Could you check a few things on this model? Use its own coordinates, in mm. Face numbers are marked on the shaded views. A direction names the side the tool comes from. Give positions to 0.01 mm unless a question says otherwise; leave off trailing zeros. Loops run counter-clockwise (first coordinate to the right, second up) from the corner with the lowest first, then second, coordinate; pieces in that order, holes last.
1. Imagine slicing it at A-A (z = 7.5). List the corners of the cut face in (x, y) for me, plus the area to 3 significant figures.
2. For the marked faces 1, 2, 3 and 4, which set-ups out of +Z, -Z, +X, -X, +Y, -Y let a thin tool reach every point of the face, with its end or its side?
3. Imagine slicing it at B-B (x = 7.5). List the corners of the cut face in (y, z) for me.
4. Thinking about a two-plate mould opening in X: for the marked faces 5, 6 and 7, which applies, +X half, -X half, draft (parallel to the pull), parting line (faces both ways), or undercut?
5. I need wall thicknesses on line 1 along Y through (x, z) = (-0.75, 7.25); line 2 along Y through (x, z) = (8.5, 1.5); line 3 along Y through (x, z) = (-6, 3.25). Which ranges of each line are inside material? Lowest first, please.
6. Imagine slicing it at C-C (x = 10). List the corners of the cut face in (y, z) for me, plus the area to 4 significant figures.
7. Imagine slicing it at D-D (z = 5.5). List the corners of the cut face in (x, y) for me.
8. For P1, Ø1.5, axis at y = 4, z = 6, coming from the -X side; P2, Ø3, axis at x = 9, y = 25, coming from the +Z side; P3, Ø1.2, axis at x = -5, y = 5, coming from the +Z side, each with a flat end and sliding along its axis, tell me the tip position at first contact or that it passes through.
```python
from build123d import *

# Parameters (mm, degrees)
SKETCH1_W           = 24
SKETCH1_H           = 19.5
BOSS_EXTRUDE1_DEPTH = 3
SKETCH3_W           = 19
SKETCH3_H           = 4.5
BOSS_EXTRUDE2_DEPTH = 1.5
SKETCH4_W           = 19
SKETCH4_H           = 6.5
BOSS_EXTRUDE3_DEPTH = 1.5
CUT_EXTRUDE1_DEPTH  = 1.5
SKETCH6_W           = 24
SKETCH6_H           = 3
BOSS_EXTRUDE4_DEPTH = 29.5
SKETCH7_W           = 4.5
SKETCH7_H           = 4.5
CUT_EXTRUDE2_DEPTH  = 39.373167709
CHAMFER1_SIZE       = 3


with BuildPart() as part:
    # Sketch1 → Boss-Extrude1 (new body)
    with BuildSketch(Plane(origin=(0, 0, 0), x_dir=(1, 0, 0), z_dir=(0, 1, 0))):
        Rectangle(SKETCH1_W, SKETCH1_H)
    extrude(amount=BOSS_EXTRUDE1_DEPTH)

    # Sketch3 → Boss-Extrude2 (add)
    with BuildSketch(Plane(origin=(0, 3, 0), x_dir=(1, 0, 0), z_dir=(0, 1, 0))):
        with Locations((0, -4.8)):
            Rectangle(SKETCH3_W, SKETCH3_H)
    extrude(amount=BOSS_EXTRUDE2_DEPTH)

    # Sketch4 → Boss-Extrude3 (add)
    with BuildSketch(Plane(origin=(0, 4.5, 0), x_dir=(1, 0, 0), z_dir=(0, 1, 0))):
        with Locations((0, -4.8)):
            Rectangle(SKETCH4_W, SKETCH4_H)
    extrude(amount=BOSS_EXTRUDE3_DEPTH)

    # Sketch5 → Cut-Extrude1 (cut)
    with BuildSketch(Plane(origin=(0, 6, 0), x_dir=(1, 0, 0), z_dir=(0, 1, 0))):
        Polygon((0, -2.8), (0.75, -1.55), (-0.75, -1.55), align=None)
        Polygon((0, -6.8), (0.75, -8.05), (-0.75, -8.05), align=None)
    extrude(amount=-CUT_EXTRUDE1_DEPTH, mode=Mode.SUBTRACT)

    # Sketch6 → Boss-Extrude4 (add)
    with BuildSketch(Plane(origin=(0, 3, 0), x_dir=(1, 0, 0), z_dir=(0, 1, 0))):
        with Locations((0, 8.25)):
            Rectangle(SKETCH6_W, SKETCH6_H)
    extrude(amount=BOSS_EXTRUDE4_DEPTH)

    # Sketch7 → Cut-Extrude2 (cut, through all)
    with BuildSketch(Plane.XY.offset(-6.75)):
        with Locations((-6.45, 27.25)):
            Rectangle(SKETCH7_W, SKETCH7_H)
        with Locations((-6.45, 14.35)):
            Rectangle(SKETCH7_W, SKETCH7_H)
        with Locations((6.45, 14.35)):
            Rectangle(SKETCH7_W, SKETCH7_H)
        with Locations((6.45, 27.25)):
            Rectangle(SKETCH7_W, SKETCH7_H)
        Polygon((-2.474873734, 20.8), (0, 23.274873734), (2.474873734, 20.8), (0, 18.325126266), align=None)
    extrude(amount=-CUT_EXTRUDE2_DEPTH, mode=Mode.SUBTRACT)

    # Chamfer1
    chamfer1_edges = [part.edges().sort_by_distance(p)[0] for p in [
        (0, 3, -6.75),
    ]]
    chamfer(chamfer1_edges, length=CHAMFER1_SIZE)


solid = part.part
```
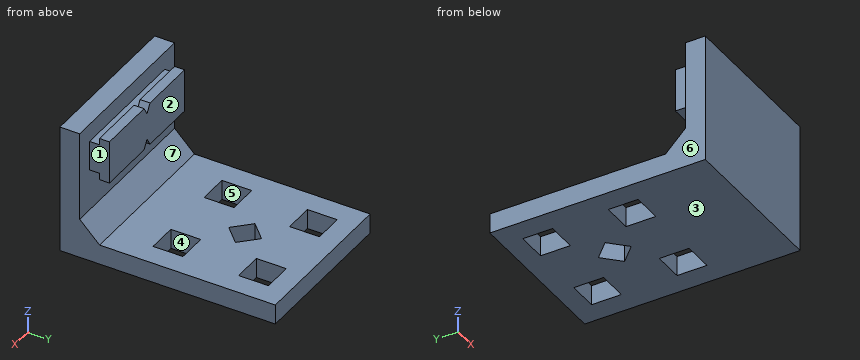
Derived:
1. outline: (-12, 0) - (12, 0) - (12, 3) - (-12, 3) - close; (-9.5, 4.5) - (-0.42, 4.5) - (-0.42, 6) - (-9.5, 6) - close; (0.42, 4.5) - (9.5, 4.5) - (9.5, 6) - (0.42, 6) - close
1. area: 99.2 mm2
2. face 1: +Z, +X, +Y
2. face 2: +Z, +X, -X, +Y
2. face 3: -Z, +X, -X, +Y, -Y
2. face 4: +Z, -Z
3. outline: (0, -9.75) - (12.1, -9.75) - (12.1, -6.75) - (6, -6.75) - (3, -3.75) - (3, 2.55) - (4.5, 2.55) - (4.5, 1.55) - (6, 1.55) - (6, 8.05) - (4.5, 8.05) - (4.5, 7.05) - (3, 7.05) - (3, 9.75) - (0, 9.75) - close; (16.6, -9.75) - (25, -9.75) - (25, -6.75) - (16.6, -6.75) - close; (29.5, -9.75) - (32.5, -9.75) - (32.5, -6.75) - (29.5, -6.75) - close
4. face 5: undercut
4. face 6: -X half
4. face 7: draft
5. line 1: y = 0 to 3, 4.5 to 6
5. line 2: y = 0 to 3
5. line 3: y = 0 to 6
6. outline: (0, -9.75) - (32.5, -9.75) - (32.5, -6.75) - (6, -6.75) - (3, -3.75) - (3, 9.75) - (0, 9.75) - close
6. area: 151.5 mm2
7. outline: (-12, 0) - (12, 0) - (12, 3) - (9.5, 3) - (9.5, 6) - (-9.5, 6) - (-9.5, 3) - (-12, 3) - close
8. P1: stops at x = -9.5
8. P2: stops at z = -6.75
8. P3: stops at z = 8.05
